```python
from build123d import *

# Parameters (mm, degrees)
BOSS_EXTRUDE1_DEPTH          = 38.1
CHAMFER1_SIZE                = 11.43
CHAMFER1_SIZE_2              = 19.797340731
F_3_8_0_375_DIAMETER_HOLE1_D = 9.525


with BuildPart() as part:
    # Sketch1 → Boss-Extrude1 (new body)
    with BuildSketch(Plane.XY):
        with BuildLine():
            Line((0, 0), (50.8, 0))
            Line((50.8, 0), (50.8, 15.875))
            Line((50.8, 15.875), (16.51, 15.875))
            Line((16.51, 15.875), (16.51, 25.4))
            Line((16.51, 25.4), (0, 25.4))
            ThreePointArc((0, 25.4), (12.7, 12.7), (0, 0))
        make_face()
    extrude(amount=BOSS_EXTRUDE1_DEPTH)

    # Chamfer1
    # the kernel refuses this chamfer: 19.797340731, 11.43 mm, written as the material it takes off along each edge
    with BuildSketch(Plane(origin=(50.8, 0, -51.217418184), x_dir=(-0.9983227437537926, -0.05789386240267138, 0), z_dir=(0, 0, 1))) as chamfer1_piece_1:
        Polygon((CHAMFER1_SIZE * 0.998322743754, -CHAMFER1_SIZE * 0.0578938624027), (-CHAMFER1_SIZE_2 * 0.0578938624012, -CHAMFER1_SIZE_2 * 0.998322743729), (0, 0), align=None)
    extrude(amount=140.534836368, mode=Mode.SUBTRACT)

    # 3/8 (0.375) Diameter Hole1 (through all)
    with Locations(Plane(origin=(0, 25.4, 0), x_dir=(1, 0, 0), z_dir=(0, 1, 0))):
        with Locations((27.939997923, -19.05)):
            Hole(F_3_8_0_375_DIAMETER_HOLE1_D / 2)


solid = part.part
```
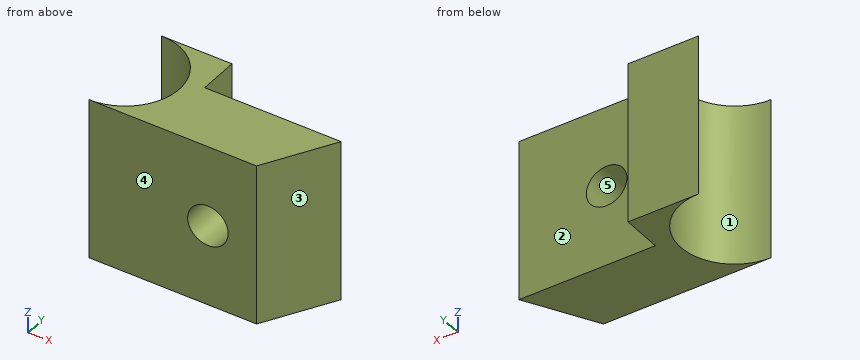
Geometry check sheet. Reference: the model listing, model coordinates, mm. Face numbers are marked on the shaded views. A direction names the side the tool comes from. Coordinates: 2 decimals unless noted, no trailing zeros. Order: outer loops, then holes, each group sorted by start corner. A loop starts at its lowest first (then second) coordinate and runs counter-clockwise, first axis right, second up.
Item 1: Depth check by flat-ended pin: pin 1 (6 mm diameter, centred on y = 16, z = 34, fed in from -X); pin 2 (1.5 mm diameter, centred on y = 3.5, z = 21.5, fed in from -X); pin 3 (1.5 mm diameter, centred on y = 12.5, z = 17, fed in from -X). Enter the tip coordinate at first touch or a pass-through.
Item 2: Section check B-B (x = 7). Enter the section's corners in (y, z), plus the area to 3 significant figures.
Item 3: Section check A-A (z = 19.05). Enter the section's corners in (x, y) (1 decimal), plus the area to 3 significant figures.
Item 4: Section check D-D (z = 26). Enter the section's corners in (x, y) (3 decimals).
Item 5: Tool access check on the marked faces 1 and 2. Record the directions out of +Z, -Z, +X, -X, +Y, -Y that give a thin tool (end or side, any length) a straight path to the whole face; none if there is none.
Item 6: Scan lines: line 1 along Y through (x, z) = (38.5, 8) (3 decimals); line 2 along Y through (x, z) = (9, 20.5); line 3 along Z through (x, y) = (24, 12). Record each from-to range of solid material in increasing order.
Item 7: Mould release check, pull along X, two halves, no side actions. Record for the marked faces 3, 4 and 5: released by +X, released by -X, zero draft, split by the parting line, or undercut.
Check sheet entries:
1. pin 1: stops at x = 11.03
1. pin 2: stops at x = 7.89
1. pin 3: stops at x = 12.66
2. outline: (0, 0) - (2.1, 0) - (2.1, 38.1) - (0, 38.1) - close; (23.3, 0) - (25.4, 0) - (25.4, 38.1) - (23.3, 38.1) - close
2. area: 160 mm2
3. outline: (0, 0) - (23.2, 0) - (23.2, 15.9) - (16.5, 15.9) - (16.5, 25.4) - (0, 25.4) arc R12.7 cw to start; (32.7, 0) - (39.4, 0) - (48.5, 15.9) - (32.7, 15.9) - close
3. area: 450 mm2
4. outline: (0, 0) - (39.37, 0) - (48.535, 15.875) - (16.51, 15.875) - (16.51, 25.4) - (0, 25.4) arc R12.7 cw to start
5. face 1: +Z, -Z, -X
5. face 2: +Z, -Z, +X, +Y
6. line 1: y = 0 to 15.875
6. line 2: y = 0 to 3.74, 21.66 to 25.4
6. line 3: z = 0 to 16.37, 21.73 to 38.1
7. face 3: released by +X
7. face 4: zero draft
7. face 5: undercut
